```python
from build123d import *

# Parameters (mm, degrees)
SKETCH1_W           = 460.375
SKETCH1_H           = 600.075
SKETCH1_W_2         = 409.575
SKETCH1_H_2         = 549.275
BOSS_EXTRUDE1_DEPTH = 617.22
SKETCH3_W           = 566.42
SKETCH3_H           = 549.275
CUT_EXTRUDE1_DEPTH  = 828.978611889
CUT_EXTRUDE2_REACH  = 955.867
SKETCH4_W           = 295.91
SKETCH4_H           = 409.575


with BuildPart() as part:
    # Sketch1 → Boss-Extrude1 (new body)
    with BuildSketch(Plane(origin=(0, 0, 0), x_dir=(0, 0, -1), z_dir=(1, 0, 0))):
        with Locations((-180.678434066, 4.335482901)):
            Rectangle(SKETCH1_W, SKETCH1_H)
        with Locations((-180.678434066, 4.335482901)):
            Rectangle(SKETCH1_W_2, SKETCH1_H_2, mode=Mode.SUBTRACT)
    extrude(amount=-BOSS_EXTRUDE1_DEPTH)

    # Sketch3 → Cut-Extrude1 (cut, through all)
    with BuildSketch(Plane.XY.offset(410.865934066)):
        with Locations((-308.61, 4.335482901)):
            Rectangle(SKETCH3_W, SKETCH3_H)
    extrude(amount=-CUT_EXTRUDE1_DEPTH, mode=Mode.SUBTRACT)

    # Sketch4 → Cut-Extrude2 (cut, up to next)
    with BuildSketch(Plane(origin=(0, 304.372982901, 0), x_dir=(1, 0, 0), z_dir=(0, 1, 0)), mode=Mode.PRIVATE) as cut_extrude2_sk1:
        with Locations((-469.265, -180.678434066)):
            Rectangle(SKETCH4_W, SKETCH4_H)
    cut_extrude2_tool1 = extrude(cut_extrude2_sk1.sketch, amount=-CUT_EXTRUDE2_REACH, mode=Mode.PRIVATE) & part.part
    # Sketch4 → Cut-Extrude2 (cut, up to next)
    with BuildSketch(Plane(origin=(0, 304.372982901, 0), x_dir=(1, 0, 0), z_dir=(0, 1, 0)), mode=Mode.PRIVATE) as cut_extrude2_sk2:
        with Locations((-147.955, -180.678434066)):
            Rectangle(SKETCH4_W, SKETCH4_H)
    cut_extrude2_tool2 = extrude(cut_extrude2_sk2.sketch, amount=-CUT_EXTRUDE2_REACH, mode=Mode.PRIVATE) & part.part
    add(cut_extrude2_tool1.solids().sort_by_distance((-469.265, 304.372983, 180.678434))[0], mode=Mode.SUBTRACT)
    add(cut_extrude2_tool2.solids().sort_by_distance((-147.955, 304.372983, 180.678434))[0], mode=Mode.SUBTRACT)


solid = part.part
```
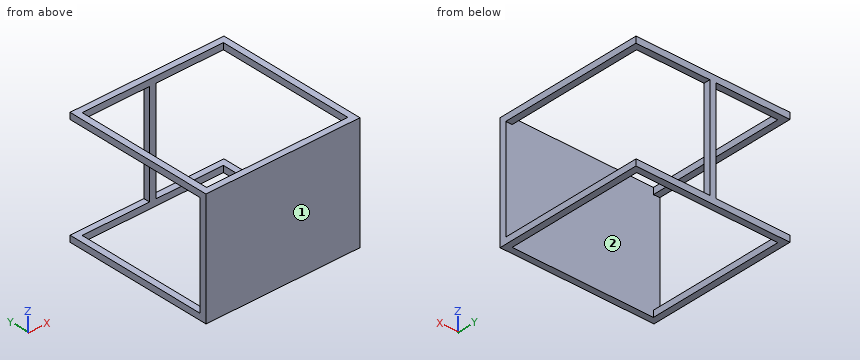
Here's how the part is built. I have some questions about the finished solid (model axes, mm). Face numbers are marked on the shaded views. Give positions to 0.01 mm unless a question says otherwise; leave off trailing zeros. Loops run counter-clockwise (first coordinate to the right, second up) from the corner with the lowest first, then second, coordinate; pieces in that order, holes last. Notation, with made-up numbers: M -16.75,-14.5 L -11.75,-14.5 A25 cw -11.75,0.5 Z; hole C -13,51.5 d1. An arc over 180 degrees is marked long. Put each result on its own line as item: value. Start each with the question number.
(1) Will these pins go through, and if not, where does the flat tip stop? pin 1 Ø20.5 at (y, z) = (297, 222.5) entering from -X; pin 2 Ø3 at (x, z) = (-332, 199) entering from +Y; pin 3 Ø7.5 at (y, z) = (292.5, 141) entering from +X.
(2) I want a section at A-A on z = 87. Please give me the cut outline in (x, y).
(3) I need wall thicknesses on line 1 along X through (y, z) = (-182, -28); line 2 along Y through (x, z) = (-183, 321). Which ranges of each line are inside material? Lowest first, please. Write a range as [from, to].
(4) I want a section at B-B on x = -198.5. Please give me the cut outline in (y, z).
(5) I want a section at C-C on y = 225.5. Please give me the cut outline in (x, z), then the cut area to 3 significant figures.
(6) If we mould it in two halves opening along Y, with no side actions, what happens to the marked faces 1 and 2? For each: +Y half, -Y half, draft (parallel to the pull), parting line (faces both ways), or undercut.
Answer block:
1. pin 1: x = -321.31
1. pin 2: y = -270.3
1. pin 3: x = -295.91
2. outline: M -617.22,-295.7 L 0,-295.7 L 0,-270.3 L -617.22,-270.3 Z; M -321.31,278.97 L -295.91,278.97 L -295.91,304.37 L -321.31,304.37 Z
3. line 1: [-617.22, -591.82], [-25.4, 0]
3. line 2: [-295.7, -270.3]
4. outline: M -295.7,-49.51 L -270.3,-49.51 L -270.3,410.87 L -295.7,410.87 Z; M 278.97,-49.51 L 304.37,-49.51 L 304.37,-24.11 L 278.97,-24.11 Z; M 278.97,385.47 L 304.37,385.47 L 304.37,410.87 L 278.97,410.87 Z
5. outline: M -617.22,-49.51 L -591.82,-49.51 L -591.82,-24.11 L -617.22,-24.11 Z; M -617.22,385.47 L -591.82,385.47 L -591.82,410.87 L -617.22,410.87 Z; M -25.4,-49.51 L 0,-49.51 L 0,-24.11 L -25.4,-24.11 Z; M -25.4,385.47 L 0,385.47 L 0,410.87 L -25.4,410.87 Z
5. area: 2,580 mm^2
6. face 1: -Y half
6. face 2: undercut
